The listing builds one solid part. Answer for the finished solid, in the listing's coordinates (mm). Give positions to 0.01 mm unless a question says otherwise; leave off trailing zeros. Write each loop counter-clockwise with the first axis right and the second up, starting at its lowest first coordinate (ties: lowest second). Pieces come first, ordered by that corner, then holes. Notation, with made-up numbers: (46, 86) - (53, 86) arc R10 ccw to (53, 105) - close; hole circle Ø2 at (-23, 20.25). An arc over 180 degrees is marked (long way). Return JSON: item names as keys, results as strings.
from build123d import *

# Parameters (mm, degrees)
SKETCH_1_W          = 340
SKETCH_1_H          = 520
EXTRUDE_1_DEPTH     = 5
SKETCH_2_W          = 20.5
SKETCH_2_H          = 41
CUT_EXTRUDE_1_DEPTH = 622.309101816
SKETCH_3_W          = 20.5
SKETCH_3_H          = 41
CUT_EXTRUDE_2_DEPTH = 15


with BuildPart() as part:
    # 스케치1 → 보스-돌출1 (new body)
    with BuildSketch(Plane(origin=(0, 0, 0), x_dir=(1, 0, 0), z_dir=(0, 1, 0))):
        with Locations((170, 260)):
            Rectangle(SKETCH_1_W, SKETCH_1_H)
    extrude(amount=EXTRUDE_1_DEPTH)

    # 스케치2 → 컷-돌출1 (cut, through all)
    with BuildSketch(Plane(origin=(0, 5, 0), x_dir=(1, 0, 0), z_dir=(0, 1, 0))):
        with Locations((329.75, 499.5)):
            Rectangle(SKETCH_2_W, SKETCH_2_H)
        with Locations((329.75, 20.5)):
            Rectangle(SKETCH_2_W, SKETCH_2_H)
        with Locations((10.25, 20.5)):
            Rectangle(SKETCH_2_W, SKETCH_2_H)
        with Locations((10.25, 499.5)):
            Rectangle(SKETCH_2_W, SKETCH_2_H)
    extrude(amount=-CUT_EXTRUDE_1_DEPTH, mode=Mode.SUBTRACT)

    # 스케치3 → 컷-돌출2 (cut)
    with BuildSketch(Plane(origin=(0, 5, 0), x_dir=(1, 0, 0), z_dir=(0, 1, 0))):
        with Locations((329.75, 210.5)):
            Rectangle(SKETCH_3_W, SKETCH_3_H)
        with Locations((10.25, 210.5)):
            Rectangle(SKETCH_3_W, SKETCH_3_H)
    extrude(amount=-CUT_EXTRUDE_2_DEPTH, mode=Mode.SUBTRACT)


solid = part.part
Item 1: A cutting plane is placed at A-A on y = 3. Determine the outline of the cut face in (x, z), then the cut area to 3 significant figures.
Answer below:
{"outline": "(0, -479) - (20.5, -479) - (20.5, -520) - (319.5, -520) - (319.5, -479) - (340, -479) - (340, -231) - (319.5, -231) - (319.5, -190) - (340, -190) - (340, -41) - (319.5, -41) - (319.5, 0) - (20.5, 0) - (20.5, -41) - (0, -41) - (0, -190) - (20.5, -190) - (20.5, -231) - (0, -231) - close", "area": "172,000 mm²"}
Item 2: Consider L1, parallel to X at y = 3.65, z = -29. Determine where the line is inside the solid, lowest interval first.
Answer below:
{"L1": "x = 20.5 to 319.5"}
Item 3: Flat-ended cylindrical pins translate along their axes: P1, Ø2.5, axis at x = 10.5, y = 3, coming from the -Z side; P2, Ø1.5, axis at x = 7, y = 2.5, coming from the +Z side; P3, Ø1.5, axis at y = 3.5, z = -215.5, coming from the +X side. Find the tip coordinate at first contact, or state that the pin passes through.
Answer below:
{"P1": "stops at z = -479", "P2": "stops at z = -41", "P3": "stops at x = 319.5"}
